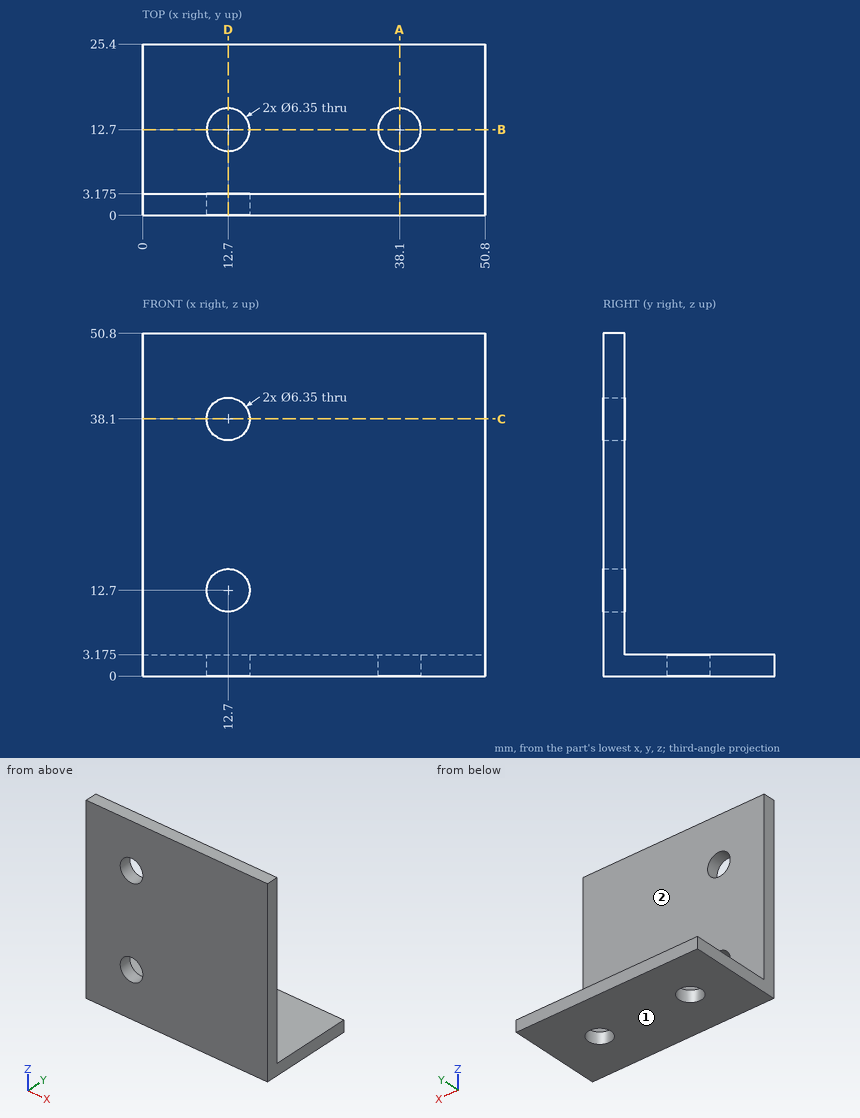
Can you work these out from the drawing? Everything is in mm from the part's minimum corner. A direction names the side the tool comes from. Round coordinates to 2 decimals unless told otherwise and drop trailing zeros. Loops run counter-clockwise (first coordinate to the right, second up) from the corner with the lowest first, then second, coordinate; pieces in that order, holes last. Notation, with made-up numbers: (19.25, -38) - (23.25, -38) arc R23 cw to (23.25, -10) - close; hole circle Ø5 at (89.5, -13.75). An arc over 180 degrees is marked (long way). Answer in a Markdown table with one row per item. Add a question column.
Q1. I want a section at B-B on y = 12.7. List the corners of the cut face in (x, z) for me (3 decimals).
Q2. Which directions (+Z, -Z, +X, -X, +Y, -Y) give clear straight access to the entire face, cutting with the end or side of a thin tool? Please do the marked faces 1 and 2.
Q3. I want a section at A-A on x = 38.1. List the corners of the cut face in (y, z) for me (3 decimals).
Q4. I need wall thicknesses on L1, parallel to Z at x = 12.7, y = 1.4 (3 decimals); L2, parallel to Y at x = 38, z = 1; L3, parallel to X at y = 2, z = 38.1 (3 decimals). Which ranges of each line are inside material? Lowest first, please.
Q5. I want a section at C-C on z = 38.1. List the corners of the cut face in (x, y) for me (3 decimals), and give its area (3 significant figures).
Q6. I want a section at D-D on x = 12.7. List the corners of the cut face in (y, z) for me (3 decimals).
Q7. For pin 1 Ø14.5 at (x, z) = (16, 22.5) entering from +Y (3 decimals); pin 2 Ø8 at (y, z) = (6, 23) entering from +X; pin 3 Ø5.5 at (x, z) = (12.7, 38.1) entering from +Y; pin 4 Ø7.5 at (x, y) = (12.7, 12.7) entering from +Z (3 decimals), each with a flat end and sliding along its axis, tell me the tip position at first contact or that it passes through.
A:
| question | item | result |
|---|---|---|
| 1 | outline | (0, 0) - (9.525, 0) - (9.525, 3.175) - (0, 3.175) - close; (15.875, 0) - (34.925, 0) - (34.925, 3.175) - (15.875, 3.175) - close; (41.275, 0) - (50.8, 0) - (50.8, 3.175) - (41.275, 3.175) - close |
| 2 | face 1 | -Z, +X, -X, +Y, -Y |
| 2 | face 2 | +Z, +X, -X, +Y |
| 3 | outline | (0, 0) - (9.525, 0) - (9.525, 3.175) - (3.175, 3.175) - (3.175, 50.8) - (0, 50.8) - close; (15.875, 0) - (25.4, 0) - (25.4, 3.175) - (15.875, 3.175) - close |
| 4 | L1 | 0 to 9.525, 15.875 to 34.925, 41.275 to 50.8 |
| 4 | L2 | 0 to 9.53, 15.87 to 25.4 |
| 4 | L3 | 0 to 9.525, 15.875 to 50.8 |
| 5 | outline | (0, 0) - (9.525, 0) - (9.525, 3.175) - (0, 3.175) - close; (15.875, 0) - (50.8, 0) - (50.8, 3.175) - (15.875, 3.175) - close |
| 5 | area | 141 mm^2 |
| 6 | outline | (0, 0) - (9.525, 0) - (9.525, 3.175) - (3.175, 3.175) - (3.175, 9.525) - (0, 9.525) - close; (0, 15.875) - (3.175, 15.875) - (3.175, 34.925) - (0, 34.925) - close; (0, 41.275) - (3.175, 41.275) - (3.175, 50.8) - (0, 50.8) - close; (15.875, 0) - (25.4, 0) - (25.4, 3.175) - (15.875, 3.175) - close |
| 7 | pin 1 | y = 3.175 |
| 7 | pin 2 | x = 50.8 |
| 7 | pin 3 | through |
| 7 | pin 4 | z = 3.175 |
